from build123d import *

# Parameters (mm, degrees)
BOSS_EXTRU_1_DEPTH      = 3
ESQUISSE2_R             = 1.25
ENL_V_MAT_EXTRU_1_DEPTH = 6.8
ESQUISSE3_W             = 6
ESQUISSE3_H             = 3
BOSS_EXTRU_2_DEPTH      = 8
ESQUISSE6_W             = 5
ESQUISSE6_H             = 6
BOSS_EXTRU_4_DEPTH      = 5
ENL_V_MAT_EXTRU_3_DEPTH = 7
CONG_2_R                = 0.5
CONG_3_R                = 2
CONG_4_R                = 1
ENL_V_MAT_EXTRU_4_DEPTH = 7


with BuildPart() as part:
    # Esquisse1 → Boss.-Extru.1 (new body, symmetric)
    with BuildSketch(Plane.XY):
        Polygon((-6, 0), (-2.4, 0), (-2.4, -2.8), (2.4, -2.8), (2.4, 0), (6, 0), (6, 3), (-6, 3), align=None)
    extrude(amount=BOSS_EXTRU_1_DEPTH, both=True)

    # Esquisse2 → Enlèv. mat.-Extru.1 (cut, through all)
    with BuildSketch(Plane(origin=(0, 3, 0), x_dir=(1, 0, 0), z_dir=(0, 1, 0))):
        Circle(ESQUISSE2_R)
    extrude(amount=-ENL_V_MAT_EXTRU_1_DEPTH, mode=Mode.SUBTRACT)

    # Esquisse3 → Boss.-Extru.2 (add)
    with BuildSketch(Plane.ZY.offset(6)):
        with Locations((0, 1.5)):
            Rectangle(ESQUISSE3_W, ESQUISSE3_H)
    extrude(amount=BOSS_EXTRU_2_DEPTH)

    # Esquisse6 → Boss.-Extru.4 (add)
    with BuildSketch(Plane.XZ):
        with Locations((-11.5, 0)):
            Rectangle(ESQUISSE6_W, ESQUISSE6_H)
    extrude(amount=BOSS_EXTRU_4_DEPTH)

    # Esquisse7 → Enlèv. mat.-Extru.3 (cut, through all)
    with BuildSketch(Plane.XY.offset(3)):
        Polygon((-14, 0.2), (-12.4988893, -2.4), (-14, -5), align=None)
    extrude(amount=-ENL_V_MAT_EXTRU_3_DEPTH, mode=Mode.SUBTRACT)

    # Congé2
    cong_2_edges = [part.edges().sort_by_distance(p)[0] for p in [
        (6, 0, 0),
        (2.4, -2.8, 0),
        (-2.4, -2.8, 0),
        (6, 3, 0),
        (-14, 3, 0),
        (-14, -5, 0),
        (-9, -5, 0),
        (-14, 0.2, 0),
    ]]
    fillet(cong_2_edges, radius=CONG_2_R)

    # Congé3
    cong_3_edges = [part.edges().sort_by_distance(p)[0] for p in [
        (-9, 0, 0),
    ]]
    fillet(cong_3_edges, radius=CONG_3_R)

    # Congé4
    cong_4_edges = [part.edges().sort_by_distance(p)[0] for p in [
        (-12.4988893, -2.4, 0),
    ]]
    fillet(cong_4_edges, radius=CONG_4_R)

    # Esquisse9 → Enlèv. mat.-Extru.4 (cut, through all)
    with BuildSketch(Plane(origin=(0, 0, -3), x_dir=(-1, 0, 0), z_dir=(0, 0, -1))):
        with BuildLine():
            Line((-4.279385242, 0), (-2.4, -0.684040287))
            ThreePointArc((-2.4, -0.684040287), (-2.997672477, 0.597672477), (-4.279385242, 0))
        make_face()
        with BuildLine():
            Line((4.279385242, 0), (2.4, -0.684040287))
            ThreePointArc((2.4, -0.684040287), (2.997672477, 0.597672477), (4.279385242, 0))
        make_face()
    extrude(amount=-ENL_V_MAT_EXTRU_4_DEPTH, mode=Mode.SUBTRACT)


solid = part.part
The listing builds one solid part. Answer for the finished solid, in the listing's coordinates (mm). A direction names the side the tool comes from. Round coordinates to 2 decimals unless told otherwise and drop trailing zeros. Order: outer loops, then holes, each group sorted by start corner. A loop starts at its lowest first (then second) coordinate and runs counter-clockwise, first axis right, second up. Notation, with made-up numbers: (-37.75, 73) -> (-15.75, 73) arc R16 ccw to (-15.75, 83) -> close; hole circle Ø4 at (76, 15). An arc over 180 degrees is marked (long way). Write each question's results on one line, items separated by ' | '. Start each with the question number.
Q1. Find section D-D (y = 1.75). Determine the outline of the cut face in (x, z), then the cut area to 3 significant figures.
Q2. Find section A-A (x = 0). Determine the outline of the cut face in (y, z).
Q3. Each of these flat-tipped pins is pushed along its axis until it touches: pin 1 (2 mm diameter, centred on x = -5.5, z = -1, fed in from -Y); pin 2 (1 mm diameter, centred on x = -0.5, z = 1, fed in from -Y); pin 3 (3 mm diameter, centred on y = -3, z = -1, fed in from -X); pin 4 (2 mm diameter, centred on x = 0, z = 0, fed in from +Y). Where does it stop, or does it pass through?
Q4. The mould has two halves that part along X. Classify faces 4 (the cylindrical face through (-8.43, -0.6, 0.04)), 5 (the flat face through (-13.172, -3.566, 0.042)), 6 (the flat face through (5, 0, 0)): pulls with the +X half, pulls with the -X half, needs draft (parallel to the pull), parting line crosses it, or undercut.
Q5. Find section B-B (z = 0). Determine the outline of the cut face in (x, y), then the cut area to 3 significant figures.
Q6. Find section C-C (y = -1). Determine the outline of the cut face in (x, z).
Q7. Which of the six approach directions +Z, -Z, +X, -X, +Y, -Y give full straight-line access (tool end or side, diameter ignored) to faces 1 (the flat face through (-6, 0, 0)), 2 (the flat face through (-13.37, -0.89, 0.04)), 3 (the flat face through (-0.4, -2.8, 1.4))?
Q8. Straight lines are drawn through the part: probe 1 along Z at (x, y) = (0, 0.8); probe 2 along X at (y, z) = (1.65, 0); probe 3 along X at (y, z) = (0.15, 0). For each, find the intervals that lie inside material, in ascending order. Write a range as from..to.
Worked answers:
1) outline: (-14, -3) -> (6, -3) -> (6, 3) -> (-14, 3) -> close; hole circle Ø2.5 at (0, 0) | area: 115 mm2
2) outline: (-2.8, -3) -> (3, -3) -> (3, -1.25) -> (-2.8, -1.25) -> close; (-2.8, 1.25) -> (3, 1.25) -> (3, 3) -> (-2.8, 3) -> close
3) pin 1: stops at y = 0 | pin 2: stops at y = -2.8 | pin 3: stops at x = -13.63 | pin 4: passes through
4) face 4: undercut | face 5: pulls with the -X half | face 6: needs draft
5) outline: (-14, 0.33) arc R0.5 ccw to (-13.93, 0.08) -> (-12.79, -1.9) arc R1 cw to (-12.79, -2.9) -> (-13.57, -4.25) arc R0.5 ccw to (-13.13, -5) -> (-9.5, -5) arc R0.5 ccw to (-9, -4.5) -> (-9, -2) arc R2 cw to (-7, 0) -> (-4.28, 0) arc R1 cw to (-2.4, -0.68) -> (-2.4, -2.3) arc R0.5 ccw to (-1.9, -2.8) -> (-1.25, -2.8) -> (-1.25, 3) -> (-13.5, 3) arc R0.5 ccw to (-14, 2.5) -> close; (1.25, -2.8) -> (1.9, -2.8) arc R0.5 ccw to (2.4, -2.3) -> (2.4, -0.68) arc R1 cw to (4.28, 0) -> (5.5, 0) arc R0.5 ccw to (6, 0.5) -> (6, 2.5) arc R0.5 ccw to (5.5, 3) -> (1.25, 3) -> close | area: 78.6 mm2
6) outline: (-13.31, -3) -> (-8.73, -3) -> (-8.73, 3) -> (-13.31, 3) -> close; (-2.4, -3) -> (2.4, -3) -> (2.4, 3) -> (-2.4, 3) -> close; hole circle Ø2.5 at (0, 0)
7) face 1: +Z, -Z, -Y | face 2: +Z, -Z, -X | face 3: +Z, -Z, +X, -Y
8) probe 1: z = -3..-1.25, 1.25..3 | probe 2: x = -14..-1.25, 1.25..6 | probe 3: x = -13.96..-4.21, -2.47..-1.25, 1.25..2.47, 4.21..5.86
